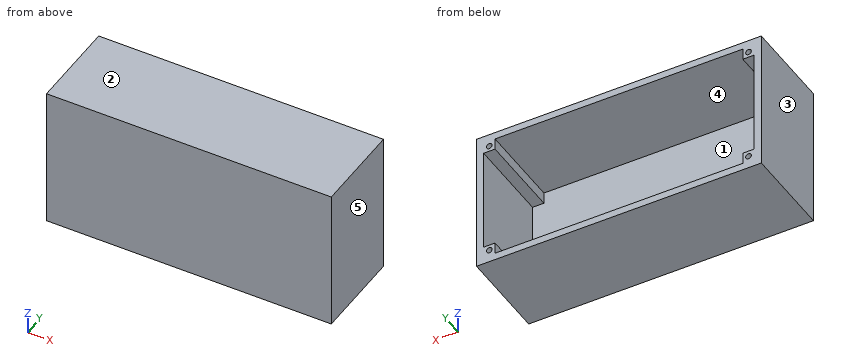
from build123d import *

# Parameters (mm, degrees)
SKETCH1_W           = 100
SKETCH1_H           = 50
BOSS_EXTRUDE1_DEPTH = 2
SKETCH3_W           = 100
SKETCH3_H           = 50
SKETCH3_R           = 1
BOSS_EXTRUDE2_DEPTH = 30


with BuildPart() as part:
    # Sketch1 → Boss-Extrude1 (new body)
    with BuildSketch(Plane(origin=(0, 0, 0), x_dir=(1, 0, 0), z_dir=(0, 1, 0))):
        with Locations((50, 25)):
            Rectangle(SKETCH1_W, SKETCH1_H)
    extrude(amount=BOSS_EXTRUDE1_DEPTH)

    # Sketch3 → Boss-Extrude2 (add)
    with BuildSketch(Plane(origin=(0, 2, 0), x_dir=(1, 0, 0), z_dir=(0, 1, 0))):
        with Locations((50, 25)):
            Rectangle(SKETCH3_W, SKETCH3_H)
        with Locations(Location((4.5, 45.5, 0), (0, 0, 270))):
            Circle(SKETCH3_R, mode=Mode.SUBTRACT)
        with Locations(Location((95.5, 45.5, 0), (0, 0, 270))):
            Circle(SKETCH3_R, mode=Mode.SUBTRACT)
        with Locations(Location((95.5, 4.5, 0), (0, 0, 270))):
            Circle(SKETCH3_R, mode=Mode.SUBTRACT)
        with Locations(Location((4.5, 4.5, 0), (0, 0, 270))):
            Circle(SKETCH3_R, mode=Mode.SUBTRACT)
        Polygon((6.5, 47.5), (93.5, 47.5), (93.5, 43.5), (97.5, 43.5), (97.5, 6.5), (93.5, 6.5), (93.5, 2.5), (6.5, 2.5), (6.5, 6.5), (2.5, 6.5), (2.5, 43.5), (6.5, 43.5), align=None, mode=Mode.SUBTRACT)
    extrude(amount=BOSS_EXTRUDE2_DEPTH)


solid = part.part
Geometry: final body of the model. Coordinates: model frame, mm. Face numbers are marked on the shaded views. A direction names the side the tool comes from. Round coordinates to 2 decimals unless told otherwise and drop trailing zeros. Loops run counter-clockwise (first coordinate to the right, second up) from the corner with the lowest first, then second, coordinate; pieces in that order, holes last. Notation, with made-up numbers: M 53,50 L 86,50 A30 cw 86,88 Z; hole C -14.5,12 d7. An arc over 180 degrees is marked long. Put each result on its own line as item: value. Start each with the question number.
(1) Contact query for a flat-ended pin moving along its axis: pin 1 Ø1.5 at (x, z) = (72.5, -34.5) entering from +Y. Output: stop coordinate, or through.
(2) Draft query along Z for the marked faces 1, 2 and 3. Return one class per face: +Z half, -Z half, draft (parallel to the pull), parting line (faces both ways), or undercut.
(3) Section query A-A (y = 3.5). Return loops of the section in (x, z), then the cut area to 3 significant figures.
(4) Set-up query: the marked faces 4 and 5. Return all of +Z, -Z, +X, -X, +Y, -Y with unobstructed straight access to the full face (end or side cutting, diameter ignored); none if empty.
(5) Material intervals for line 1 along X through (y, z) = (20.5, -45.5); line 2 along Z through (x, y) = (95.5, 23.75); line 3 along Z through (x, y) = (61, 20.5), sorted ascending. Write a range as [from, to].
(6) Section query D-D (z = -12). Return loops of the section in (x, y), then the cut area to 3 significant figures.
(7) Section query B-B (z = -4.5). Return loops of the section in (x, y).
(8) Section query C-C (x = 72.5). Return loops of the section in (y, z).
Findings below:
1. pin 1: stops at y = 2
2. face 1: undercut
2. face 2: +Z half
2. face 3: draft
3. outline: M 0,-50 L 100,-50 L 100,0 L 0,0 Z; hole M 2.5,-43.5 L 6.5,-43.5 L 6.5,-47.5 L 93.5,-47.5 L 93.5,-43.5 L 97.5,-43.5 L 97.5,-6.5 L 93.5,-6.5 L 93.5,-2.5 L 6.5,-2.5 L 6.5,-6.5 L 2.5,-6.5 Z; hole C 4.5,-45.5 d2; hole C 4.5,-4.5 d2; hole C 95.5,-45.5 d2; hole C 95.5,-4.5 d2
3. area: 776 mm2
4. face 4: +Y
4. face 5: +Z, -Z, +X, +Y, -Y
5. line 1: x = [0, 3.5], [5.5, 6.5], [93.5, 94.5], [96.5, 100]
5. line 2: z = [-50, -46.5], [-44.5, -43.5], [-6.5, -5.5], [-3.5, 0]
5. line 3: z = [-50, -47.5], [-2.5, 0]
6. outline: M 0,0 L 100,0 L 100,32 L 97.5,32 L 97.5,2 L 2.5,2 L 2.5,32 L 0,32 Z
6. area: 350 mm2
7. outline: M 0,0 L 100,0 L 100,32 L 96.5,32 L 96.5,2 L 94.5,2 L 94.5,32 L 93.5,32 L 93.5,2 L 6.5,2 L 6.5,32 L 5.5,32 L 5.5,2 L 3.5,2 L 3.5,32 L 0,32 Z
8. outline: M 0,-50 L 32,-50 L 32,-47.5 L 2,-47.5 L 2,-2.5 L 32,-2.5 L 32,0 L 0,0 Z
